from build123d import *

# Parameters (mm, degrees)
SKETCH1_W           = 164.1
SKETCH1_H           = 174.745
SKETCH1_R           = 1.4732
SKETCH1_W_2         = 56.35
SKETCH1_H_2         = 56.35
BOSS_EXTRUDE1_DEPTH = 1.5875
FILLET1_R           = 1


with BuildPart() as part:
    # Sketch1 → Boss-Extrude1 (new body)
    with BuildSketch(Plane.XY):
        with Locations((82.55, -87.3725)):
            Rectangle(SKETCH1_W, SKETCH1_H)
        with Locations((82.55, -152.3725)):
            Circle(SKETCH1_R, mode=Mode.SUBTRACT)
        with Locations((82.55, -87.3725)):
            Rectangle(SKETCH1_W_2, SKETCH1_H_2, mode=Mode.SUBTRACT)
        with Locations((82.55, -22.3725)):
            Circle(SKETCH1_R, mode=Mode.SUBTRACT)
        with BuildLine():
            Line((82.55, -5.4375), (80.434372699, -5.4375))
            ThreePointArc((80.434372699, -5.4375), (75.6625, -3.85), (80.434372699, -2.2625))
            Line((80.434372699, -2.2625), (82.55, -2.2625))
            ThreePointArc((82.55, -2.2625), (84.1375, -3.85), (82.55, -5.4375))
        make_face(mode=Mode.SUBTRACT)
        with BuildLine():
            Line((16.934372699, -168.395), (19.05, -168.395))
            ThreePointArc((19.05, -168.395), (20.6375, -169.9825), (19.05, -171.57))
            Line((19.05, -171.57), (16.934372699, -171.57))
            ThreePointArc((16.934372699, -171.57), (12.1625, -169.9825), (16.934372699, -168.395))
        make_face(mode=Mode.SUBTRACT)
        with BuildLine():
            Line((7.409372699, -151.9325), (9.525, -151.9325))
            ThreePointArc((9.525, -151.9325), (11.1125, -153.52), (9.525, -155.1075))
            Line((9.525, -155.1075), (7.409372699, -155.1075))
            ThreePointArc((7.409372699, -155.1075), (2.6375, -153.52), (7.409372699, -151.9325))
        make_face(mode=Mode.SUBTRACT)
        with BuildLine():
            Line((42.334372699, -168.395), (44.45, -168.395))
            ThreePointArc((44.45, -168.395), (46.0375, -169.9825), (44.45, -171.57))
            Line((44.45, -171.57), (42.334372699, -171.57))
            ThreePointArc((42.334372699, -171.57), (37.5625, -169.9825), (42.334372699, -168.395))
        make_face(mode=Mode.SUBTRACT)
        with BuildLine():
            Line((67.734372699, -168.395), (69.85, -168.395))
            ThreePointArc((69.85, -168.395), (71.4375, -169.9825), (69.85, -171.57))
            Line((69.85, -171.57), (67.734372699, -171.57))
            ThreePointArc((67.734372699, -171.57), (62.9625, -169.9825), (67.734372699, -168.395))
        make_face(mode=Mode.SUBTRACT)
        with BuildLine():
            Line((7.409372699, -126.5325), (9.525, -126.5325))
            ThreePointArc((9.525, -126.5325), (11.1125, -128.12), (9.525, -129.7075))
            Line((9.525, -129.7075), (7.409372699, -129.7075))
            ThreePointArc((7.409372699, -129.7075), (2.6375, -128.12), (7.409372699, -126.5325))
        make_face(mode=Mode.SUBTRACT)
        with Locations((26.258348754, -119.8725)):
            Circle(SKETCH1_R, mode=Mode.SUBTRACT)
        with BuildLine():
            Line((7.409372699, -101.1325), (9.525, -101.1325))
            ThreePointArc((9.525, -101.1325), (11.1125, -102.72), (9.525, -104.3075))
            Line((9.525, -104.3075), (7.409372699, -104.3075))
            ThreePointArc((7.409372699, -104.3075), (2.6375, -102.72), (7.409372699, -101.1325))
        make_face(mode=Mode.SUBTRACT)
        with BuildLine():
            Line((7.409372699, -75.7325), (9.525, -75.7325))
            ThreePointArc((9.525, -75.7325), (11.1125, -77.32), (9.525, -78.9075))
            Line((9.525, -78.9075), (7.409372699, -78.9075))
            ThreePointArc((7.409372699, -78.9075), (2.6375, -77.32), (7.409372699, -75.7325))
        make_face(mode=Mode.SUBTRACT)
        with BuildLine():
            Line((7.409372699, -50.3325), (9.525, -50.3325))
            ThreePointArc((9.525, -50.3325), (11.1125, -51.92), (9.525, -53.5075))
            Line((9.525, -53.5075), (7.409372699, -53.5075))
            ThreePointArc((7.409372699, -53.5075), (2.6375, -51.92), (7.409372699, -50.3325))
        make_face(mode=Mode.SUBTRACT)
        with Locations((26.258348754, -54.8725)):
            Circle(SKETCH1_R, mode=Mode.SUBTRACT)
        with BuildLine():
            Line((7.409372699, -24.9325), (9.525, -24.9325))
            ThreePointArc((9.525, -24.9325), (11.1125, -26.52), (9.525, -28.1075))
            Line((9.525, -28.1075), (7.409372699, -28.1075))
            ThreePointArc((7.409372699, -28.1075), (2.6375, -26.52), (7.409372699, -24.9325))
        make_face(mode=Mode.SUBTRACT)
        with BuildLine():
            Line((7.409372699, -8.1), (9.525, -8.1))
            ThreePointArc((9.525, -8.1), (11.1125, -9.6875), (9.525, -11.275))
            Line((9.525, -11.275), (7.409372699, -11.275))
            ThreePointArc((7.409372699, -11.275), (2.6375, -9.6875), (7.409372699, -8.1))
        make_face(mode=Mode.SUBTRACT)
        with BuildLine():
            Line((29.634372699, -2.2625), (31.75, -2.2625))
            ThreePointArc((31.75, -2.2625), (33.3375, -3.85), (31.75, -5.4375))
            Line((31.75, -5.4375), (29.634372699, -5.4375))
            ThreePointArc((29.634372699, -5.4375), (24.8625, -3.85), (29.634372699, -2.2625))
        make_face(mode=Mode.SUBTRACT)
        with BuildLine():
            Line((55.034372699, -2.2625), (57.15, -2.2625))
            ThreePointArc((57.15, -2.2625), (58.7375, -3.85), (57.15, -5.4375))
            Line((57.15, -5.4375), (55.034372699, -5.4375))
            ThreePointArc((55.034372699, -5.4375), (50.2625, -3.85), (55.034372699, -2.2625))
        make_face(mode=Mode.SUBTRACT)
        with BuildLine():
            ThreePointArc((161.925, -8.1), (163.5125, -9.6875), (161.925, -11.275))
            Line((161.925, -11.275), (159.809372699, -11.275))
            ThreePointArc((159.809372699, -11.275), (155.0375, -9.6875), (159.809372699, -8.1))
            Line((159.809372699, -8.1), (161.925, -8.1))
        make_face(mode=Mode.SUBTRACT)
        with BuildLine():
            Line((93.134372699, -168.395), (95.25, -168.395))
            ThreePointArc((95.25, -168.395), (96.8375, -169.9825), (95.25, -171.57))
            Line((95.25, -171.57), (93.134372699, -171.57))
            ThreePointArc((93.134372699, -171.57), (88.3625, -169.9825), (93.134372699, -168.395))
        make_face(mode=Mode.SUBTRACT)
        with BuildLine():
            Line((118.534372699, -168.395), (120.65, -168.395))
            ThreePointArc((120.65, -168.395), (122.2375, -169.9825), (120.65, -171.57))
            Line((120.65, -171.57), (118.534372699, -171.57))
            ThreePointArc((118.534372699, -171.57), (113.7625, -169.9825), (118.534372699, -168.395))
        make_face(mode=Mode.SUBTRACT)
        with BuildLine():
            Line((143.934372699, -168.395), (146.05, -168.395))
            ThreePointArc((146.05, -168.395), (147.6375, -169.9825), (146.05, -171.57))
            Line((146.05, -171.57), (143.934372699, -171.57))
            ThreePointArc((143.934372699, -171.57), (139.1625, -169.9825), (143.934372699, -168.395))
        make_face(mode=Mode.SUBTRACT)
        with BuildLine():
            Line((159.809372699, -151.9325), (161.925, -151.9325))
            ThreePointArc((161.925, -151.9325), (163.5125, -153.52), (161.925, -155.1075))
            Line((161.925, -155.1075), (159.809372699, -155.1075))
            ThreePointArc((159.809372699, -155.1075), (155.0375, -153.52), (159.809372699, -151.9325))
        make_face(mode=Mode.SUBTRACT)
        with Locations((138.841651246, -119.8725)):
            Circle(SKETCH1_R, mode=Mode.SUBTRACT)
        with BuildLine():
            Line((159.809372699, -126.5325), (161.925, -126.5325))
            ThreePointArc((161.925, -126.5325), (163.5125, -128.12), (161.925, -129.7075))
            Line((161.925, -129.7075), (159.809372699, -129.7075))
            ThreePointArc((159.809372699, -129.7075), (155.0375, -128.12), (159.809372699, -126.5325))
        make_face(mode=Mode.SUBTRACT)
        with BuildLine():
            Line((159.809372699, -101.1325), (161.925, -101.1325))
            ThreePointArc((161.925, -101.1325), (163.5125, -102.72), (161.925, -104.3075))
            Line((161.925, -104.3075), (159.809372699, -104.3075))
            ThreePointArc((159.809372699, -104.3075), (155.0375, -102.72), (159.809372699, -101.1325))
        make_face(mode=Mode.SUBTRACT)
        with BuildLine():
            Line((159.809372699, -75.7325), (161.925, -75.7325))
            ThreePointArc((161.925, -75.7325), (163.047532015, -78.442532015), (160.3375, -77.32))
            ThreePointArc((160.3375, -77.32), (155.172995809, -78.156521771), (159.809372699, -75.7325))
        make_face(mode=Mode.SUBTRACT)
        with Locations((138.841651246, -54.8725)):
            Circle(SKETCH1_R, mode=Mode.SUBTRACT)
        with BuildLine():
            Line((159.809372699, -50.3325), (161.925, -50.3325))
            ThreePointArc((161.925, -50.3325), (163.5125, -51.92), (161.925, -53.5075))
            Line((161.925, -53.5075), (159.809372699, -53.5075))
            ThreePointArc((159.809372699, -53.5075), (155.0375, -51.92), (159.809372699, -50.3325))
        make_face(mode=Mode.SUBTRACT)
        with BuildLine():
            Line((105.834372699, -2.2625), (107.95, -2.2625))
            ThreePointArc((107.95, -2.2625), (109.5375, -3.85), (107.95, -5.4375))
            Line((107.95, -5.4375), (105.834372699, -5.4375))
            ThreePointArc((105.834372699, -5.4375), (101.0625, -3.85), (105.834372699, -2.2625))
        make_face(mode=Mode.SUBTRACT)
        with BuildLine():
            Line((159.809372699, -24.9325), (161.925, -24.9325))
            ThreePointArc((161.925, -24.9325), (163.5125, -26.52), (161.925, -28.1075))
            Line((161.925, -28.1075), (159.809372699, -28.1075))
            ThreePointArc((159.809372699, -28.1075), (155.0375, -26.52), (159.809372699, -24.9325))
        make_face(mode=Mode.SUBTRACT)
        with BuildLine():
            Line((131.234372699, -2.2625), (133.35, -2.2625))
            ThreePointArc((133.35, -2.2625), (134.9375, -3.85), (133.35, -5.4375))
            Line((133.35, -5.4375), (131.234372699, -5.4375))
            ThreePointArc((131.234372699, -5.4375), (126.4625, -3.85), (131.234372699, -2.2625))
        make_face(mode=Mode.SUBTRACT)
    extrude(amount=BOSS_EXTRUDE1_DEPTH)

    # Fillet1
    fillet1_edges = [part.edges().sort_by_distance(p)[0] for p in [
        (0.5, -174.745, 0.79375),
        (0.5, 0, 0.79375),
        (164.6, 0, 0.79375),
        (164.6, -174.745, 0.79375),
    ]]
    fillet(fillet1_edges, radius=FILLET1_R)


solid = part.part
Part model, mm, in its own coordinate system. Give positions to 0.01 mm unless a question says otherwise; leave off trailing zeros.
(1) Pin check, flat tip, straight feed: pin 1 (6 mm diameter, centred on x = 157.69, y = -9.69, fed in from -Z). Stop position of the tip, or through.
Return value:
pin 1: stops at z = 0
(2) Drill centre lines: line 1 along Y through (x, z) = (69, 1.3) (1 decimal); line 2 along Y through (x, z) = (139, 0.3) (3 decimals); line 3 along X through (y, z) = (-93, 0.6) (3 decimals). Where is each one in solid material? Low to high.
Return value:
line 1: y = -174.7 to -171.6, -168.4 to -115.5, -59.2 to 0
line 2: y = -174.745 to -121.337, -118.408 to -56.337, -53.408 to 0
line 3: x = 0.5 to 54.375, 110.725 to 164.6
(3) Band-saw the part on A-A (z = 0.85). Count the separate pieces of the cut face and the enclosed holes in it, and give its area (3 significant figures).
Return value:
separate pieces: 1
enclosed holes: 32
area: 24,700 mm2
(4) Pull direction X, two halves, no side cores. Call faces 1 (the flat face through (118, -86, 1.588)), 2 (the cylindrical face through (113.764, -170.075, 0.783)): pulls with the +X half, pulls with the -X half, needs draft (parallel to the pull), parting line crosses it, or undercut.
Return value:
face 1: needs draft
face 2: undercut
